Check sheet for the modelled part. Datum: model origin and axes. Units: mm. A direction names the side the tool comes from. Give positions to 0.01 mm unless a question says otherwise; leave off trailing zeros. Loops run counter-clockwise (first coordinate to the right, second up) from the corner with the lowest first, then second, coordinate; pieces in that order, holes last. Notation, with made-up numbers: (-14, 66) - (-7, 66) arc R20 ccw to (-7, 95) - close; hole circle Ø8 at (-22.75, 48). An arc over 180 degrees is marked (long way). Use one line per item in the form item = value.
from build123d import *
from build123d.topology import SkipClean

# Parameters (mm, degrees)
CROQUIS1_W                = 5
CROQUIS1_H                = 30
SALIENTE_EXTRUIR1_DEPTH   = 19.1
SALIENTE_EXTRUIR1_2_DEPTH = 19.1
CROQUIS2_W                = 30
CROQUIS2_H                = 5
CROQUIS2_H_2              = 20
SALIENTE_EXTRUIR2_DEPTH   = 24
CORTAR_EXTRUIR1_REACH     = 56.173
CROQUIS3_R                = 2.5
CROQUIS4_R                = 4.65
CORTAR_EXTRUIR2_DEPTH     = 2.5
REDONDEO1_R               = 10
CORTAR_EXTRUIR8_REACH     = 48.271
CROQUIS12_R               = 2.5
REDONDEO2_DEPTH           = 29.797959071
REDONDEO2_START           = 4.55
REDONDEO2_2_DEPTH         = 6.55
REDONDEO2_START_2         = 7.549995607
REDONDEO2_3_DEPTH         = 6.550004393
CORTAR_EXTRUIR10_DEPTH    = 3
CROQUIS15_W               = 11
CROQUIS15_H               = 6
CORTAR_EXTRUIR11_DEPTH    = 34
CORTAR_EXTRUIR14_REACH    = 48.271
CROQUIS17_R               = 2.5
CROQUIS18_W               = 11
CROQUIS18_H               = 8.1
CORTAR_EXTRUIR15_DEPTH    = 34
SALIENTE_EXTRUIR3_REACH   = 56.173
CORTAR_EXTRUIR16_REACH    = 47.889
CROQUIS20_W               = 24
CROQUIS20_H               = 10


with BuildPart() as part:
    # Croquis1 → Saliente-Extruir1 (new body)
    with BuildSketch(Plane(origin=(0, 0, 0), x_dir=(1, 0, 0), z_dir=(0, 1, 0))):
        with Locations((2.5, -15)):
            Rectangle(CROQUIS1_W, CROQUIS1_H)
    extrude(amount=SALIENTE_EXTRUIR1_DEPTH)



with BuildPart() as body_2:
    # Croquis1 → Saliente-Extruir1 2 (new body)
    with BuildSketch(Plane(origin=(0, 0, 0), x_dir=(1, 0, 0), z_dir=(0, 1, 0))):
        with Locations((-26.5, -15)):
            Rectangle(CROQUIS1_W, CROQUIS1_H)
    extrude(amount=SALIENTE_EXTRUIR1_2_DEPTH)


with BuildPart() as part_1:
    add(part.part)

    add(body_2.part)  # Saliente-Extruir2 merges body 2
    # Croquis2 → Saliente-Extruir2 (add)
    with BuildSketch(Plane.ZY):
        with Locations((15, 16.6)):
            Rectangle(CROQUIS2_W, CROQUIS2_H)
        with Locations((15, -5.45)):
            Rectangle(CROQUIS2_W, CROQUIS2_H_2)
    extrude(amount=SALIENTE_EXTRUIR2_DEPTH)

    # Croquis3 → Cortar-Extruir1 (cut, up to next)
    with BuildSketch(Plane(origin=(0, 19.1, 0), x_dir=(1, 0, 0), z_dir=(0, 1, 0)), mode=Mode.PRIVATE) as cortar_extruir1_sk1:
        with Locations(Location((-12, -21, 0), (0, 0, 270))):
            Circle(CROQUIS3_R)
    cortar_extruir1_tool1 = extrude(cortar_extruir1_sk1.sketch, amount=-CORTAR_EXTRUIR1_REACH, mode=Mode.PRIVATE) & part_1.part
    add(cortar_extruir1_tool1.solids().sort_by_distance((-12, 19.1, 21))[0], mode=Mode.SUBTRACT)

    # Croquis4 → Cortar-Extruir2 (cut)
    with BuildSketch(Plane(origin=(0, 19.1, 0), x_dir=(1, 0, 0), z_dir=(0, 1, 0))):
        with Locations(Location((-12, -21, 0), (0, 0, 270))):
            Circle(CROQUIS4_R)
    extrude(amount=-CORTAR_EXTRUIR2_DEPTH, mode=Mode.SUBTRACT)

    # Redondeo1
    # the kernel refuses this fillet: 10 mm, written as the material it takes off along each edge
    with BuildSketch(Plane(origin=(-29, -25, 30), x_dir=(1, 0, 0), z_dir=(0, 1, 0)), Plane(origin=(5, -25, 30), x_dir=(0, 0, -1), z_dir=(0, 1, 0))) as redondeo1_piece_1:
        with BuildLine():
            CenterArc((REDONDEO1_R, REDONDEO1_R), REDONDEO1_R, 180, 90)
            Line((0, REDONDEO1_R), (0, 0))
            Line((0, 0), (REDONDEO1_R, 0))
        make_face()
    extrude(amount=69.1, mode=Mode.SUBTRACT)

    # Cortar-Extruir8: up to this face of the body (flat: up to its plane)
    cortar_extruir8_end = Plane(part_1.part.faces().sort_by_distance((-12, -15.45, 14.911465184))[0])
    # Croquis12 → Cortar-Extruir8 (cut, up to the picked face)
    with BuildSketch(Plane(origin=(0, 4.55, 0), x_dir=(1, 0, 0), z_dir=(0, 1, 0)), mode=Mode.PRIVATE) as cortar_extruir8_sk1:
        with Locations(Location((-24, -6, 0), (0, 0, 270))):
            Circle(CROQUIS12_R)
    cortar_extruir8_tool1 = split(extrude(cortar_extruir8_sk1.sketch, amount=-CORTAR_EXTRUIR8_REACH, mode=Mode.PRIVATE), bisect_by=cortar_extruir8_end, keep=Keep.BOTH, mode=Mode.PRIVATE)
    # Croquis12 → Cortar-Extruir8 (cut, up to the picked face)
    with BuildSketch(Plane(origin=(0, 4.55, 0), x_dir=(1, 0, 0), z_dir=(0, 1, 0)), mode=Mode.PRIVATE) as cortar_extruir8_sk2:
        with Locations(Location((0, -6, 0), (0, 0, 270))):
            Circle(CROQUIS12_R)
    cortar_extruir8_tool2 = split(extrude(cortar_extruir8_sk2.sketch, amount=-CORTAR_EXTRUIR8_REACH, mode=Mode.PRIVATE), bisect_by=cortar_extruir8_end, keep=Keep.BOTH, mode=Mode.PRIVATE)
    add(cortar_extruir8_tool1.solids().sort_by(Axis((-24, 4.55, 6), (0, -1, 0)))[0], mode=Mode.SUBTRACT)
    add(cortar_extruir8_tool2.solids().sort_by(Axis((0, 4.55, 6), (0, -1, 0)))[0], mode=Mode.SUBTRACT)

    # Redondeo2: read off the stored shape, not the designer's step
    # Redondeo2 outline → Redondeo2 (add)
    with BuildSketch(Plane.XY):
        with BuildLine():
            Line((-24, 14.1), (-24, 11.1))
            ThreePointArc((-24, 11.1), (-23.121320344, 13.221320344), (-21, 14.1))
            Line((-21, 14.1), (-24, 14.1))
        make_face()
        with BuildLine():
            ThreePointArc((-21, 4.55), (-23.121320344, 5.428679656), (-24, 7.55))
            Line((-24, 7.55), (-24, 4.55))
            Line((-24, 4.55), (-21, 4.55))
        make_face()
        with BuildLine():
            Line((0, 14.1), (-3, 14.1))
            ThreePointArc((-3, 14.1), (-0.878679656, 13.221320344), (0, 11.1))
            Line((0, 11.1), (0, 14.1))
        make_face()
        with BuildLine():
            ThreePointArc((0, 7.55), (-0.878679656, 5.428679656), (-3, 4.55))
            Line((-3, 4.55), (0, 4.55))
            Line((0, 4.55), (0, 7.55))
        make_face()
    extrude(amount=REDONDEO2_DEPTH)

    # Redondeo2 2 outline → Redondeo2 2 (cut)
    with BuildSketch(Plane(origin=(0, 0, 0), x_dir=(1, 0, 0), z_dir=(0, 1, 0)).offset(REDONDEO2_START)):
        with BuildLine():
            ThreePointArc((-24, -8.5), (-21.5, -6), (-24, -3.5))
            Line((-24, -3.5), (-24, -8.5))
        make_face()
        with BuildLine():
            ThreePointArc((-20.99999998, -29.797958975), (-22.545926263, -29.350208925), (-24, -28.660254038))
            Line((-24, -28.660254038), (-24, -29.797959071))
            Line((-24, -29.797959071), (-20.99999998, -29.797958975))
        make_face()
        with BuildLine():
            Line((0, -29.797959071), (0, -28.660254038))
            ThreePointArc((0, -28.660254038), (-1.454073737, -29.350208925), (-3.00000002, -29.797958975))
            Line((-3.00000002, -29.797958975), (0, -29.797959071))
        make_face()
        with BuildLine():
            Line((0, -8.5), (0, -3.5))
            ThreePointArc((0, -3.5), (-2.5, -6), (0, -8.5))
        make_face()
    extrude(amount=REDONDEO2_2_DEPTH, mode=Mode.SUBTRACT)

    # Redondeo2 3 outline → Redondeo2 3 (cut)
    with BuildSketch(Plane(origin=(0, 0, 0), x_dir=(1, 0, 0), z_dir=(0, 1, 0)).offset(REDONDEO2_START_2)):
        with BuildLine():
            ThreePointArc((-20.99999998, -29.797958975), (-22.545926263, -29.350208925), (-24, -28.660254038))
            Line((-24, -28.660254038), (-24, -29.797959071))
            Line((-24, -29.797959071), (-20.99999998, -29.797958975))
        make_face()
        with BuildLine():
            Line((0, -29.797959071), (0, -28.660254038))
            ThreePointArc((0, -28.660254038), (-1.454073737, -29.350208925), (-3.00000002, -29.797958975))
            Line((-3.00000002, -29.797958975), (0, -29.797959071))
        make_face()
    extrude(amount=REDONDEO2_3_DEPTH, mode=Mode.SUBTRACT)

    # Croquis14 → Cortar-Extruir10 (cut, symmetric)
    with SkipClean():  # the faces are left unmerged after this step: merging them gives an invalid solid
        with BuildSketch(Plane(origin=(0, 4.55, 0), x_dir=(1, 0, 0), z_dir=(0, 1, 0))):
            Polygon((-5.541319679, -6.117372146), (-2.669012579, -10.857609685), (2.872307099, -10.740237539), (5.541319679, -5.882627854), (2.669012579, -1.142390315), (-2.872307099, -1.259762461), align=None)
            Polygon((-18.457437416, -6), (-21.228718708, -1.2), (-26.771281292, -1.2), (-29.542562584, -6), (-26.771281292, -10.8), (-21.228718708, -10.8), align=None)
        extrude(amount=CORTAR_EXTRUIR10_DEPTH, both=True, mode=Mode.SUBTRACT)

    # Croquis15 → Cortar-Extruir11 (cut)
    with BuildSketch(Plane(origin=(5, 0, 0), x_dir=(0, 0, -1), z_dir=(1, 0, 0))):
        with Locations((-5.5, 8)):
            Rectangle(CROQUIS15_W, CROQUIS15_H)
    extrude(amount=-CORTAR_EXTRUIR11_DEPTH, mode=Mode.SUBTRACT)

    # Croquis17 → Cortar-Extruir14 (cut, up to next)
    with BuildSketch(Plane(origin=(0, 4.55, 0), x_dir=(1, 0, 0), z_dir=(0, 1, 0)), mode=Mode.PRIVATE) as cortar_extruir14_sk1:
        with Locations(Location((-12, -21, 0), (0, 0, 270))):
            Circle(CROQUIS17_R)
    cortar_extruir14_tool1 = extrude(cortar_extruir14_sk1.sketch, amount=-CORTAR_EXTRUIR14_REACH, mode=Mode.PRIVATE) & part_1.part
    add(cortar_extruir14_tool1.solids().sort_by_distance((-12, 4.55, 21))[0], mode=Mode.SUBTRACT)

    # Croquis18 → Cortar-Extruir15 (cut)
    with BuildSketch(Plane(origin=(5, 0, 0), x_dir=(0, 0, -1), z_dir=(1, 0, 0))):
        with Locations((-5.5, 15.05)):
            Rectangle(CROQUIS18_W, CROQUIS18_H)
    extrude(amount=-CORTAR_EXTRUIR15_DEPTH, mode=Mode.SUBTRACT)

    # Croquis19 → Saliente-Extruir3 (add, up to next)
    with BuildSketch(Plane(origin=(0, -15.45, 0), x_dir=(-1, 0, 0), z_dir=(0, -1, 0)), mode=Mode.PRIVATE) as saliente_extruir3_sk1:
        with BuildLine():
            Line((0, -28.660254038), (0, -8.5))
            ThreePointArc((0, -8.5), (-2.5, -6), (0, -3.5))
            Line((0, -3.5), (0, 0))
            Line((0, 0), (-5, 0))
            Line((-5, 0), (-5, -20))
            ThreePointArc((-5, -20), (-3.660254038, -25), (0, -28.660254038))
        make_face()
    saliente_extruir3_tool1 = extrude(saliente_extruir3_sk1.sketch, amount=-SALIENTE_EXTRUIR3_REACH, mode=Mode.PRIVATE) - part_1.part
    # Croquis19 → Saliente-Extruir3 (add, up to next)
    with BuildSketch(Plane(origin=(0, -15.45, 0), x_dir=(-1, 0, 0), z_dir=(0, -1, 0)), mode=Mode.PRIVATE) as saliente_extruir3_sk2:
        with BuildLine():
            Line((24, -8.5), (24, -28.660254038))
            ThreePointArc((24, -28.660254038), (27.660254038, -25), (29, -20))
            Line((29, -20), (29, 0))
            Line((29, 0), (24, 0))
            Line((24, 0), (24, -3.5))
            ThreePointArc((24, -3.5), (26.5, -6), (24, -8.5))
        make_face()
    saliente_extruir3_tool2 = extrude(saliente_extruir3_sk2.sketch, amount=-SALIENTE_EXTRUIR3_REACH, mode=Mode.PRIVATE) - part_1.part
    add(saliente_extruir3_tool1.solids().sort_by_distance((2.502598, -15.45, 13.726714))[0])
    add(saliente_extruir3_tool2.solids().sort_by_distance((-26.502598, -15.45, 13.726714))[0])

    # Croquis20 → Cortar-Extruir16 (cut, up to next)
    with BuildSketch(Plane(origin=(0, 0, 0), x_dir=(-1, 0, 0), z_dir=(0, 0, -1)), mode=Mode.PRIVATE) as cortar_extruir16_sk1:
        with Locations((12, -5.45)):
            Rectangle(CROQUIS20_W, CROQUIS20_H)
    cortar_extruir16_tool1 = extrude(cortar_extruir16_sk1.sketch, amount=-CORTAR_EXTRUIR16_REACH, mode=Mode.PRIVATE) & part_1.part
    add(cortar_extruir16_tool1.solids().sort_by_distance((-12, -5.45, 0))[0], mode=Mode.SUBTRACT)


solid = part_1.part
Item 1: Section check D-D on x = -8.5. Record the boundary of the cut face in (y, z).
Answer block:
outline = (-15.45, 0) - (-10.45, 0) - (-10.45, 30) - (-15.45, 30) - close; (-0.45, 0) - (4.55, 0) - (4.55, 30) - (-0.45, 30) - close; (14.1, 11) - (19.1, 11) - (19.1, 17.94) - (16.6, 17.94) - (16.6, 24.06) - (19.1, 24.06) - (19.1, 30) - (14.1, 30) - close
Item 2: Thickness scan on L1, parallel to X at y = 0, z = 6; L2, parallel to Y at x = -5, z = 24; L3, parallel to Y at x = -15.5, z = 4. Record the ranges inside material, lowest first.
Answer block:
L1 = -29 to -26.5, -21.5 to -2.5, 2.5 to 5
L2 = -15.45 to -10.45, -0.45 to 4.55, 14.1 to 19.1
L3 = -15.45 to -10.45, -0.45 to 4.55
Item 3: Gauge pin test, flat ends, axial feed: P1, Ø1.2, axis at x = 1, z = 9.5, coming from the +Y side; P2, Ø8, axis at x = -14.5, y = 12, coming from the -Z side; P3, Ø5.5, axis at x = -27, z = 2.5, coming from the +Y side. Record the tip position at first contact, or that the pin passes through.
Answer block:
P1 = 1.55
P2 = 11
P3 = 5
Item 4: Mould release check, pull along Z, two halves, no side actions. Record for faces 6 (the face through (-27.87, 3.3, 3.1)), 7 (the face through (-0.9, 13.24, 20.27)), 8 (the face through (-12, -13, 30)): released by +Z, released by -Z, zero draft, split by the parting line, or undercut.
Answer block:
face_6 = undercut
face_7 = zero draft
face_8 = released by +Z
Item 5: Section check A-A on x = -12. Record the boundary of the cut face in (y, z).
Answer block:
outline = (-15.45, 0) - (-10.45, 0) - (-10.45, 18.5) - (-15.45, 18.5) - close; (-15.45, 23.5) - (-10.45, 23.5) - (-10.45, 30) - (-15.45, 30) - close; (-0.45, 0) - (4.55, 0) - (4.55, 18.5) - (-0.45, 18.5) - close; (-0.45, 23.5) - (4.55, 23.5) - (4.55, 30) - (-0.45, 30) - close; (14.1, 11) - (19.1, 11) - (19.1, 16.35) - (16.6, 16.35) - (16.6, 18.5) - (14.1, 18.5) - close; (14.1, 23.5) - (16.6, 23.5) - (16.6, 25.65) - (19.1, 25.65) - (19.1, 30) - (14.1, 30) - close
Item 6: Section check B-B on y = -9. Record the boundary of the cut face in (x, z), then the cut area to 3 significant figures.
Answer block:
outline = (-29, 0) - (-24, 0) - (-24, 3.5) arc R2.5 cw to (-24, 8.5) - (-24, 28.66) arc R10 ccw to (-29, 20) - close; (0, 0) - (5, 0) - (5, 20) arc R10 ccw to (0, 28.66) - (0, 8.5) arc R2.5 cw to (0, 3.5) - close
area = 242 mm2
Item 7: Access from +Z, -Z, +X, -X, +Y, -Y to the whole of each face (thin tool, end or side, straight path). Record for faces 1 (the face through (0, 9, 20)), 2 (the face through (-13.5, 15.4, 19)), 3 (the face through (3, 5, 1)), 4 (the face through (-21.81, 4.66, 0.61)), 5 (the face through (-24, 3, 1.2)).
Answer block:
face_1 = +Z, -Z
face_2 = +Y, -Y
face_3 = -Z, +X, -X, +Y
face_4 = +Z, -Z, +Y
face_5 = +Y
